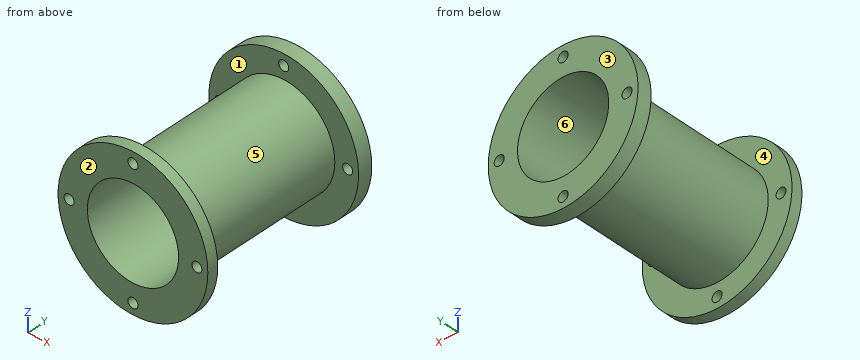
```python
from build123d import *

# Parameters (mm, degrees)
F0_R     = 41
F1_DEPTH = 8
F2_R     = 28
F3_DEPTH = 85.5
F4_R     = 41
F4_R_2   = 28
F5_DEPTH = 6
F6_R     = 25
F7_DEPTH = 99.501
F8_R     = 2.75
F9_DEPTH = 99.501


with BuildPart() as f1:
    # F0 (on Front) → F1 (new body)
    with BuildSketch(Plane.XZ):
        Circle(F0_R)
    extrude(amount=F1_DEPTH)

    # F2 (on face) → F3 (join)
    with BuildSketch(Plane.XZ.offset(8)):
        Circle(F2_R)
    extrude(amount=F3_DEPTH)

    # F4 (on face) → F5 (join)
    with BuildSketch(Plane.XZ.offset(93.5)):
        Circle(F4_R)
        Circle(F4_R_2, mode=Mode.SUBTRACT)
        Circle(F4_R_2)
    extrude(amount=F5_DEPTH)

    # F6 (on face) → F7 (cut, through all)
    with BuildSketch(Plane.XZ.offset(99.5)):
        Circle(F6_R)
    extrude(amount=-F7_DEPTH, mode=Mode.SUBTRACT)

    # F8 (on face) → F9 (cut, through all)
    with BuildSketch(Plane.XZ.offset(99.5)):
        with Locations((-35, 0)):
            Circle(F8_R)
        with Locations((0, 35)):
            Circle(F8_R)
        with Locations((35, 0)):
            Circle(F8_R)
        with Locations((0, -35)):
            Circle(F8_R)
    extrude(amount=-F9_DEPTH, mode=Mode.SUBTRACT)


solid = f1.part
```
Could you check a few things on this model? Use its own coordinates, in mm. Face numbers are marked on the shaded views. A direction names the side the tool comes from. Round coordinates to 2 decimals unless told otherwise and drop trailing zeros. Loops run counter-clockwise (first coordinate to the right, second up) from the corner with the lowest first, then second, coordinate; pieces in that order, holes last. Notation, with made-up numbers: (52, 19.25) - (78, 19.25) arc R20 cw to (78, 45.25) - close; hole circle Ø1 at (-39, -22.75). An arc over 180 degrees is marked (long way). Use CSV: the item, a comma, the result in double quotes.
Item 1: If we section it at A-A on x = 0: Count the separate pieces of the cut face and the enclosed holes in it, then the cut area to 3 significant figures.
Here are the results:
separate pieces,"6"
enclosed holes,"0"
area,"807 mm²"
Item 2: If we mould it in two halves opening along Y, with no side actions, what happens to the marked faces 3, 4, 5 and 6? For each: pulls with the +Y half, pulls with the -Y half, needs draft (parallel to the pull), parting line crosses it, or undercut.
Here are the results:
face 3,"pulls with the +Y half"
face 4,"undercut"
face 5,"undercut"
face 6,"needs draft"
Item 3: If we section it at D-D on x = 8.5: List the corners of the cut face in (y, z) for me, then the cut area to 3 significant figures.
Here are the results:
outline,"(-99.5, -40.11) - (-93.5, -40.11) - (-93.5, -26.68) - (-8, -26.68) - (-8, -40.11) - (0, -40.11) - (0, -23.51) - (-99.5, -23.51) - close; (-99.5, 23.51) - (0, 23.51) - (0, 40.11) - (-8, 40.11) - (-8, 26.68) - (-93.5, 26.68) - (-93.5, 40.11) - (-99.5, 40.11) - close"
area,"1,010 mm²"
Item 4: I need wall thicknesses on L1, parallel to Z at x = 0, y = -97.05; L2, parallel to Y at x = 0.5, z = 29.5; L3, parallel to Z at x = 35, y = -6.25. Which ranges of each line are inside material? Lowest first, please. Write a range as [from, to].
Here are the results:
L1,"z = [-41, -37.75], [-32.25, -25], [25, 32.25], [37.75, 41]"
L2,"y = [-99.5, -93.5], [-8, 0]"
L3,"z = [-21.35, -2.75], [2.75, 21.35]"
Item 5: For the marked faces 1 and 2, which set-ups out of +Z, -Z, +X, -X, +Y, -Y let a thin tool reach every point of the face, with its end or its side?
Here are the results:
face 1,"none"
face 2,"+Z, -Z, +X, -X, -Y"
Item 6: Will these pins go through, and if not, where does the flat tip stop? pin 1 (10 mm diameter, centred on x = 7, y = -13.5, fed in from -Z); pin 2 (8 mm diameter, centred on x = 8, y = -71.5, fed in from +Z); pin 3 (6 mm diameter, centred on x = -18.5, y = -57.5, fed in from -Z).
Here are the results:
pin 1,"stops at z = -27.93"
pin 2,"stops at z = 27.71"
pin 3,"stops at z = -23.32"
Item 7: If we section it at C-C on z = 21: List the corners of the cut face in (x, y) for me.
Here are the results:
outline,"(-35.21, -99.5) - (-13.56, -99.5) - (-13.56, 0) - (-35.21, 0) - (-35.21, -8) - (-18.52, -8) - (-18.52, -93.5) - (-35.21, -93.5) - close; (13.56, -99.5) - (35.21, -99.5) - (35.21, -93.5) - (18.52, -93.5) - (18.52, -8) - (35.21, -8) - (35.21, 0) - (13.56, 0) - close"
